```python
from build123d import *

# Parameters (mm, degrees)
F1_DEPTH = 50.8


with BuildPart() as f1:
    # F0 (on Front) → F1 (new body)
    with BuildSketch(Plane.XZ):
        Polygon((-30.170836, 0), (20.628821, 0), (20.623103, 25.4), (-4.770836, 25.4), (-4.770836, 36.663294), (-4.770836, 50.8), (-30.170836, 50.8), align=None)
        with BuildLine():
            Line((-4.770836, 25.4), (20.623103, 25.4))
            ThreePointArc((20.623103, 25.4), (6.733233, 28.342164), (-4.770836, 36.663294))
            Line((-4.770836, 36.663294), (-4.770836, 25.4))
        make_face()
    extrude(amount=F1_DEPTH)


solid = f1.part
```
Check sheet for the modelled part. Datum: model origin and axes. Units: mm. A direction names the side the tool comes from. Give positions to 0.01 mm unless a question says otherwise; leave off trailing zeros. Write each loop counter-clockwise with the first axis right and the second up, starting at its lowest first coordinate (ties: lowest second). Pieces come first, ordered by that corner, then holes. Notation, with made-up numbers: (10.5, 58.5) -> (33.5, 58.5) arc R20 ccw to (33.5, 78.5) -> close; hole circle Ø3 at (-2.75, -10.75). An arc over 180 degrees is marked (long way). Use CSV: the item, a comma, the result in double quotes. Start each with the question number.
Q1. Tool access check on faces 1 (the flat face through (-11, 0, 20)), 2 (the flat face through (-4.771, -25, 44)). Record the directions out of +Z, -Z, +X, -X, +Y, -Y that give a thin tool (end or side, any length) a straight path to the whole face; none if there is none.
Q2. Cross-section at C-C on x = 15. Enter the section's corners in (y, z).
Q3. Depth check by flat-ended pin: P1, Ø8, axis at y = -45, z = 26, coming from the +X side; P2, Ø5, axis at y = -7.5, z = 36.5, coming from the +X side; P3, Ø2, axis at x = -16.5, y = -14.5, coming from the -Z side; P4, Ø11.5, axis at y = -25, z = 41.5, coming from the +X side. Enter the tip coordinate at first touch or a pass-through.
Q4. Cross-section at B-B on z = 38. Enter the section's corners in (x, y).
Q5. Cross-section at A-A on y = -34. Enter the section's corners in (x, z), and give its area (3 significant figures).
Q6. Scan lines: line 1 along X through (y, z) = (-9, 14); line 2 along X through (y, z) = (-44, 48.5); line 3 along Z through (x, y) = (3.5, -5). Record each from-to range of solid material in increasing order.
Working result:
1,face 1,"+Z, -Z, +X, -X, +Y"
1,face 2,"+Z, +X, +Y, -Y"
2,outline,"(-50.8, 0) -> (0, 0) -> (0, 25.86) -> (-50.8, 25.86) -> close"
3,P1,"stops at x = 20.62"
3,P2,"stops at x = -2.08"
3,P3,"stops at z = 0"
3,P4,"stops at x = -3.91"
4,outline,"(-30.17, -50.8) -> (-4.77, -50.8) -> (-4.77, 0) -> (-30.17, 0) -> close"
5,outline,"(-30.17, 0) -> (20.63, 0) -> (20.62, 25.4) arc R34.26 cw to (-4.77, 36.66) -> (-4.77, 50.8) -> (-30.17, 50.8) -> close"
5,area,"2,020 mm^2"
6,line 1,"x = -30.17 to 20.63"
6,line 2,"x = -30.17 to -4.77"
6,line 3,"z = 0 to 29.99"
